For this review, take the finished solid that the model builds, in its own axes (mm). A direction names the side the tool comes from. Coordinates: 2 decimals unless noted, no trailing zeros. Write each loop counter-clockwise with the first axis right and the second up, starting at its lowest first coordinate (ties: lowest second). Pieces come first, ordered by that corner, then holes.
```python
from build123d import *

# Parameters (mm, degrees)
F0_W     = 40
F0_H     = 30
F0_H_2   = 10
F1_DEPTH = 3.5
F3_START = -10
F3_DEPTH = 30


with BuildPart() as f1:
    # F0 (on Front) → F1 (new body, symmetric)
    with BuildSketch(Plane.XZ):
        with Locations((-20, 0)):
            Rectangle(F0_W, F0_H)
        Polygon((0, 40.5), (0, 15), (0, -15), (0, -40.5), (10, -40.5), (10, -30.5), (10, 30.5), (10, 40.5), align=None)
        with Locations((30, 35.5)):
            Rectangle(F0_W, F0_H_2)
        with Locations((30, -35.5)):
            Rectangle(F0_W, F0_H_2)
    extrude(amount=F1_DEPTH, both=True)

    # F2 (on Right) → F3 (cut)
    with BuildSketch(Plane.YZ.offset(F3_START)):
        with BuildLine():
            ThreePointArc((-1.5329709717, 2.1), (-1.1777681167, -2.3179435418), (2.6, 0))
            ThreePointArc((2.6, 0), (2.3179435418, 1.1777681167), (1.5329709717, 2.1))
            Line((1.5329709717, 2.1), (-1.5329709717, 2.1))
        make_face()
    extrude(amount=-F3_DEPTH, mode=Mode.SUBTRACT)


solid = f1.part
```
Q1. Tool access review of faces 5 (the flat face through (-20, 0, -15)), 6 (the flat face through (0, 0, 28)), 7 (the flat face through (50, 0, 35)), 8 (the flat face through (25, 0, 40.5)), 9 (the flat face through (10, 0, 0)): name each direction out of +Z, -Z, +X, -X, +Y, -Y from which nothing blocks a thin tool from reaching the whole face with its end or side.
Ans:
face 5: -Z, -X, +Y, -Y
face 6: +Z, -X, +Y, -Y
face 7: +Z, -Z, +X, +Y, -Y
face 8: +Z, +X, -X, +Y, -Y
face 9: +X, +Y, -Y
Q2. Add section D-D (z = -21). State the section outline as (x, y) points.
Ans:
outline: (0, -3.5) - (10, -3.5) - (10, 3.5) - (0, 3.5) - close
Q3. Add section C-C (y = 0). State the section outline as (x, z) points.
Ans:
outline: (-40, -15) - (0, -15) - (0, -40.5) - (50, -40.5) - (50, -30.5) - (10, -30.5) - (10, 30.5) - (50, 30.5) - (50, 40.5) - (0, 40.5) - (0, 15) - (-40, 15) - (-40, 2.1) - (-10, 2.1) - (-10, -2.6) - (-40, -2.6) - close
Q4. For probe 1 along Z at (x, y) = (-16.5, 0); probe 2 along Z at (x, y) = (19, 3); probe 3 along X at (y, z) = (-0.75, 36), list the stretches that pass through material, from the lowest coordinate up.
Ans:
probe 1: z = -15 to -2.6, 2.1 to 15
probe 2: z = -40.5 to -30.5, 30.5 to 40.5
probe 3: x = 0 to 50
Q5. Clearance check with flat-ended pins moving along their axes: pin 1 Ø2 at (x, y) = (-8, -2) entering from -Z; pin 2 Ø2.5 at (y, z) = (0.5, 0.5) entering from -X; pin 3 Ø1 at (y, z) = (-2.5, -27.5) entering from -X. State where each tip first meets the part, or that it passes through.
Ans:
pin 1: stops at z = -15
pin 2: stops at x = -10
pin 3: stops at x = 0
Q6. Draft analysis for pull direction Y (two halves, no side actions). For faces 1 (the flat face through (1, -3.5, 3)), 2 (the flat face through (0, 0, -28)), 3 (the flat face through (-10, 0, 0)), 4 (the flat face through (-25, 0, 2.1)), state which applies: +Y half, -Y half, draft (parallel to the pull), parting line (faces both ways), or undercut.
Ans:
face 1: -Y half
face 2: draft
face 3: undercut
face 4: undercut
Q7. Add section B-B (x = -26.5). State the section outline as (y, z) points.
Ans:
outline: (-3.5, -15) - (3.5, -15) - (3.5, 15) - (-3.5, 15) - close; hole (-1.53, 2.1) arc R2.6 ccw (long way) to (1.53, 2.1) - close
Q8. Add section A-A (x = 14). State the section outline as (y, z) points.
Ans:
outline: (-3.5, -40.5) - (3.5, -40.5) - (3.5, -30.5) - (-3.5, -30.5) - close; (-3.5, 30.5) - (3.5, 30.5) - (3.5, 40.5) - (-3.5, 40.5) - close
